For this review, use the dimensioned drawing (mm, ordinates from the lowest corner) and the shaded views. Give positions to 0.01 mm unless a question says otherwise; leave off trailing zeros. Loops run counter-clockwise (first coordinate to the right, second up) from the corner with the lowest first, then second, coordinate; pieces in that order, holes last. Notation, with made-up numbers: (-3.75, 39) -> (3.25, 39) arc R16 cw to (3.25, 45) -> close; hole circle Ø4 at (88, 68.25). An arc over 180 degrees is marked (long way). Write each question's results on one line, items separated by ' | '. Start each with the question number.
Q1. Wall thickness on L1, parallel to Z at x = 20, y = 2.45; L2, parallel to Z at x = 4, y = 1.2; L3, parallel to X at y = 3.25, z = 31: over which ranges is each line inside the solid? List them lowest first. Write a range as [from, to].
Q2. We need section D-D (x = 4). Write out the cut boundary in (y, z).
Q3. We need section A-A (x = 20). Write out the cut boundary in (y, z).
Q4. We need section B-B (z = 42). Write out the cut boundary in (x, y).
Q5. Insertion check: pin 1 Ø3 at (x, z) = (11, 12) entering from +Y; pin 2 Ø2.5 at (x, z) = (20, 3) entering from -Y; pin 3 Ø3.5 at (y, z) = (1, 20) entering from +X; pin 4 Ø6 at (y, z) = (13.5, 16.5) entering from +X. Each pin has a flat end and moves straight along its axis. Give the tip position at first contact, or say it passes through.
Q6. We need section C-C (y = 1.75). Write out the cut boundary in (x, z), plus the area to 3 significant figures.
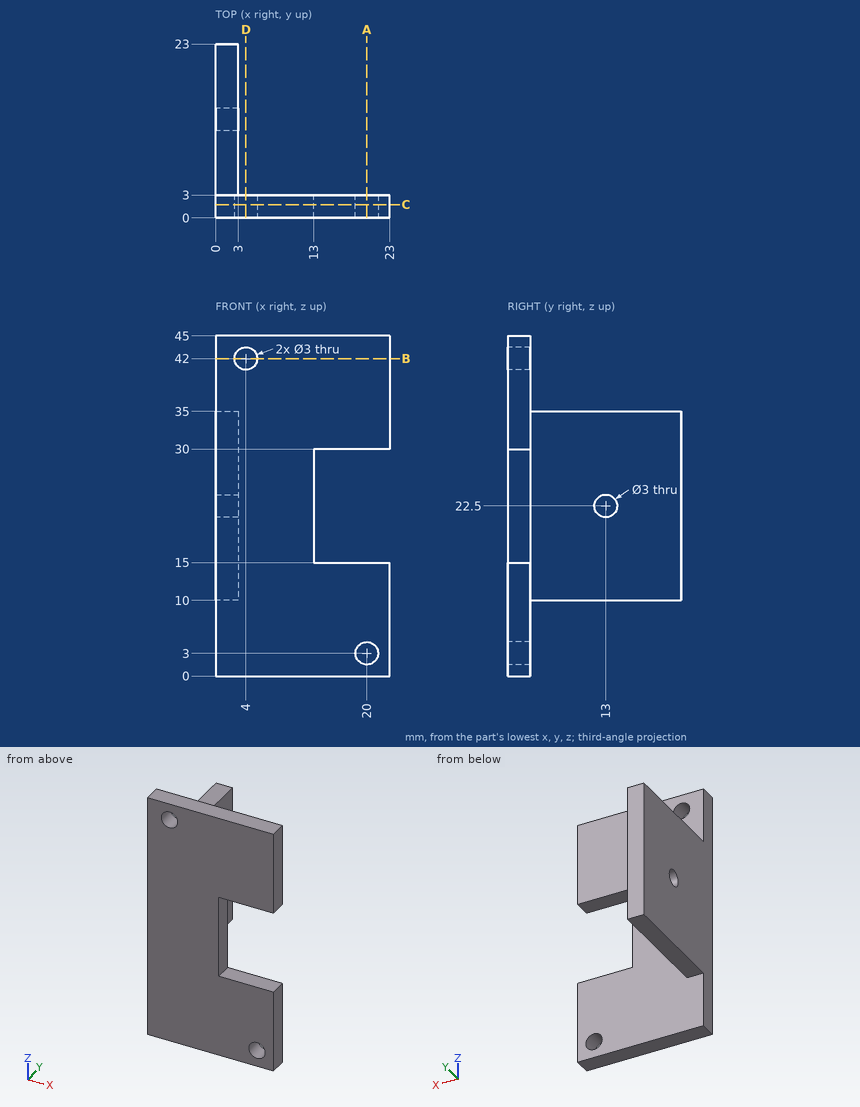
Output:
1) L1: [0, 1.5], [4.5, 15], [30, 45] | L2: [0, 40.5], [43.5, 45] | L3: [0, 3]
2) outline: (0, 0) -> (3, 0) -> (3, 40.5) -> (0, 40.5) -> close; (0, 43.5) -> (3, 43.5) -> (3, 45) -> (0, 45) -> close
3) outline: (0, 0) -> (3, 0) -> (3, 1.5) -> (0, 1.5) -> close; (0, 4.5) -> (3, 4.5) -> (3, 15) -> (0, 15) -> close; (0, 30) -> (3, 30) -> (3, 45) -> (0, 45) -> close
4) outline: (0, 0) -> (2.5, 0) -> (2.5, 3) -> (0, 3) -> close; (5.5, 0) -> (23, 0) -> (23, 3) -> (5.5, 3) -> close
5) pin 1: y = 3 | pin 2: through | pin 3: x = 13 | pin 4: x = 3
6) outline: (0, 0) -> (23, 0) -> (23, 15) -> (13, 15) -> (13, 30) -> (23, 30) -> (23, 45) -> (0, 45) -> close; hole circle Ø3 at (4, 42); hole circle Ø3 at (20, 3) | area: 871 mm2
